from build123d import *

# Parameters (mm, degrees)
F0_R     = 3
F1_DEPTH = 3


with BuildPart() as f1:
    # F0 (on Front) → F1 (new body)
    with BuildSketch(Plane.XZ):
        with BuildLine():
            ThreePointArc((5.0238306032, 7.4673372811), (2.4989245726, 8.1910870463), (0, 9))
            ThreePointArc((0, 9), (-9, 0), (0, -9))
            ThreePointArc((0, -9), (2.0891997796, -8.459259966), (4.1899294664, -7.9652050235))
            ThreePointArc((4.1899294664, -7.9652050235), (7.7041990238, -4.6524528371), (9, 0))
            ThreePointArc((9, 0), (7.944006402, 4.2299837217), (5.0238306032, 7.4673372811))
        make_face()
        Circle(F0_R, mode=Mode.SUBTRACT)
        with BuildLine():
            ThreePointArc((44.8388245261, 7.3730772224), (24.9251697087, 4.8191586202), (5.0238306032, 7.4673372811))
            ThreePointArc((5.0238306032, 7.4673372811), (7.944006402, 4.2299837217), (9, 0))
            ThreePointArc((9, 0), (7.7041990238, -4.6524528371), (4.1899294664, -7.9652050235))
            ThreePointArc((4.1899294664, -7.9652050235), (24.7899854963, -5.6356561903), (45.4138690609, -7.7438622799))
            ThreePointArc((45.4138690609, -7.7438622799), (41.0065045418, -0.3421102804), (44.8388245261, 7.3730772224))
        make_face()
        with BuildLine():
            ThreePointArc((50.2100552652, 8.9975483764), (47.5391507079, 8.1366722514), (44.8388245261, 7.3730772224))
            ThreePointArc((44.8388245261, 7.3730772224), (41.0065045418, -0.3421102804), (45.4138690609, -7.7438622799))
            ThreePointArc((45.4138690609, -7.7438622799), (47.9935464321, -8.3282112662), (50.5563037426, -8.9827905545))
            ThreePointArc((50.5563037426, -8.9827905545), (56.5576952386, -6.16414091), (59, 0))
            ThreePointArc((59, 0), (56.4377984353, 6.2892568167), (50.2100552652, 8.9975483764))
        make_face()
        with Locations((50, 0)):
            Circle(F0_R, mode=Mode.SUBTRACT)
    extrude(amount=F1_DEPTH)


solid = f1.part
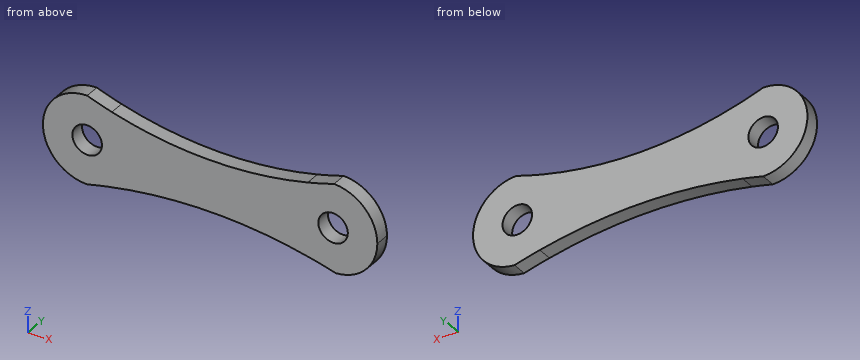
Here's how the part is built. I have some questions about the finished solid (model axes, mm). Round coordinates to 2 decimals unless told otherwise and drop trailing zeros. Write each loop counter-clockwise with the first axis right and the second up, starting at its lowest first coordinate (ties: lowest second). Pieces come first, ordered by that corner, then holes.
1. I need wall thicknesses on L1, parallel to X at y = -0.7, z = -2.25; L2, parallel to X at y = -2.2, z = -1.75; L3, parallel to Z at x = -1.5, y = -2.6. Which ranges of each line are inside material? Lowest first, please.
2. Suppose I cut it at D-D (z = -7). List the corners of the cut face in (x, y) for me.
3. Suppose I cut it at B-B (z = -2.25). List the corners of the cut face in (x, y) for me, and give its area (3 significant figures).
4. Suppose I cut it at C-C (y = -1.1). List the corners of the cut face in (x, z) for me, and give its area (3 significant figures).
5. Suppose I cut it at A-A (x = -1). List the corners of the cut face in (y, z) for me.
6. Will these pins go through, and if not, where does the flat tip stop? pin 1 Ø4 at (x, z) = (25.5, -2) entering from +Y; pin 2 Ø1.5 at (y, z) = (-2, 3) entering from -X; pin 3 Ø3.5 at (x, z) = (0, 0) entering from +Y.
Answer sheet:
1. L1: x = -8.71 to -1.98, 1.98 to 48.02, 51.98 to 58.71
1. L2: x = -8.83 to -2.44, 2.44 to 47.56, 52.44 to 58.83
1. L3: z = -8.87 to -2.6, 2.6 to 8.87
2. outline: (-5.66, -3) - (9.1, -3) - (9.1, 0) - (-5.66, 0) - close; (41.52, -3) - (55.66, -3) - (55.66, 0) - (41.52, 0) - close
3. outline: (-8.71, -3) - (-1.98, -3) - (-1.98, 0) - (-8.71, 0) - close; (1.98, -3) - (48.02, -3) - (48.02, 0) - (1.98, 0) - close; (51.98, -3) - (58.71, -3) - (58.71, 0) - (51.98, 0) - close
3. area: 178 mm2
4. outline: (0, -9) arc R96.85 cw to (50.56, -8.98) arc R9 ccw to (50.21, 9) arc R77.48 cw to (0, 9) arc R9 ccw to start; hole circle Ø6 at (0, 0); hole circle Ø6 at (50, 0)
4. area: 843 mm2
5. outline: (-3, -8.94) - (0, -8.94) - (0, -2.83) - (-3, -2.83) - close; (-3, 2.83) - (0, 2.83) - (0, 8.94) - (-3, 8.94) - close
6. pin 1: stops at y = 0
6. pin 2: stops at x = -8.71
6. pin 3: passes through
